Design review of the part built by this model. Coordinates are the model's own, in mm. A direction names the side the tool comes from. Round coordinates to 2 decimals unless told otherwise and drop trailing zeros. Order: outer loops, then holes, each group sorted by start corner. A loop starts at its lowest first (then second) coordinate and runs counter-clockwise, first axis right, second up. Notation, with made-up numbers: (-38.75, 43.5) - (1.25, 43.5) arc R19 cw to (1.25, 67.5) - close; hole circle Ø9 at (25.25, -39). An arc over 180 degrees is marked (long way). Write item = value, one per line.
from build123d import *

# Parameters (mm, degrees)
F0_W     = 6.35
F0_H     = 301.752
F1_DEPTH = 101.6
F3_DEPTH = 101.6
F5_DEPTH = 4.7625
F7_DEPTH = 4.7625
F8_W     = 127
F8_H     = 190.5
F9_DEPTH = 9.525
F11_D    = 11.1125


with BuildPart() as f1:
    # F0 (on Front) → F1 (new body, symmetric)
    with BuildSketch(Plane.XZ):
        Polygon((-19.05, -454.152), (0, -454.152), (0, 0), (-19.05, 0), (-19.05, -301.752), align=None)
        with Locations((-22.225, -150.876)):
            Rectangle(F0_W, F0_H)
    extrude(amount=F1_DEPTH, both=True)

    # F2 (on Front) → F3 (join, symmetric)
    with BuildSketch(Plane.XZ):
        Polygon((-158.75, 0), (0, 0), (298.45, 0), (298.45, 12.7), (-158.75, 12.7), align=None)
    extrude(amount=F3_DEPTH, both=True)

    # F4 (on Front) → F5 (join, symmetric)
    with BuildSketch(Plane.XZ):
        Polygon((-25.4, -127), (-25.4, 0), (-152.4, 0), (-152.4, -25.4), (-50.8, -127), align=None)
    extrude(amount=F5_DEPTH, both=True)

    # F6 (on Front) → F7 (join, symmetric)
    with BuildSketch(Plane.XZ):
        Polygon((292.1, 0), (0, 0), (0, -454.152), (25.4, -454.152), (292.1, -25.4), align=None)
    extrude(amount=F7_DEPTH, both=True)

    # F8 (on face) → F9 (join)
    with BuildSketch(Plane.XY.offset(12.7)):
        with Locations((-88.9, 0)):
            Rectangle(F8_W, F8_H)
        with Locations((228.6, 0)):
            Rectangle(F8_W, F8_H)
    extrude(amount=F9_DEPTH)

    # F11 (through all)
    with Locations(Plane.XY.offset(22.225)):
        with Locations((-127, 61.976), (-50.8, 61.976), (-127, -61.976), (-50.8, -61.976), (190.5, 61.976), (266.7, 61.976), (266.7, -61.976), (190.5, -61.976)):
            Hole(F11_D / 2)


solid = f1.part
Item 1: Take a section at D-D, the plane x = 102.5. State the section outline as (y, z) points.
Data:
outline = (-101.6, 0) - (-4.76, 0) - (-4.76, -330.2) - (4.76, -330.2) - (4.76, 0) - (101.6, 0) - (101.6, 12.7) - (-101.6, 12.7) - close
Item 2: Insertion check: P1, Ø10, axis at y = -73.5, z = -347, coming from the +X side; P2, Ø13, axis at x = 190.5, y = 61.976, coming from the -Z side; P3, Ø10.5, axis at x = 205.5, z = 19, coming from the -Y side. Each pin has a flat end and moves straight along its axis. Give the tip position at first contact, or say it passes through.
Data:
P1 = 0
P2 = 0
P3 = -95.25
Item 3: For faces 4 (the face through (-19.05, -1, -377)), 5 (the face through (-76, -4.762, -48)), 6 (the face through (194.595, 65.731, 10.957)), 7 (the face through (112, 4.762, -173)), list the 3-axis set-ups (+Z, -Z, +X, -X, +Y, -Y) from which the entire face can be reached by the end or side of a thin tool; tool diameter is ignored.
Data:
face_4 = -Z, -X, +Y, -Y
face_5 = -Z, -X, -Y
face_6 = +Z, -Z
face_7 = -Z, +X, +Y
Item 4: Take a section at B-B, the plane y = -36.5. State the section outline as (x, z) points (3 decimals).
Data:
outline = (-158.75, 0) - (-25.4, 0) - (-25.4, -301.752) - (-19.05, -301.752) - (-19.05, -454.152) - (0, -454.152) - (0, 0) - (298.45, 0) - (298.45, 12.7) - (292.1, 12.7) - (292.1, 22.225) - (165.1, 22.225) - (165.1, 12.7) - (-25.4, 12.7) - (-25.4, 22.225) - (-152.4, 22.225) - (-152.4, 12.7) - (-158.75, 12.7) - close
Item 5: Take a section at C-C, the plane z = -280. State the section outline as (x, y) points.
Data:
outline = (-25.4, -101.6) - (0, -101.6) - (0, -4.76) - (133.73, -4.76) - (133.73, 4.76) - (0, 4.76) - (0, 101.6) - (-25.4, 101.6) - close
Item 6: Take a section at A-A, the plane x = -127. Count the separate pieces of the cut face and the enclosed holes in it, and give its area (3 significant figures).
Data:
separate_pieces = 3
enclosed_holes = 0
area = 4,390 mm2
Item 7: For line 1 along Y through (x, z) = (266, 10); line 2 along Y through (x, z) = (-127, 6); line 3 along Z through (x, y) = (105, -68), list the stretches that pass through material, from the lowest coordinate up. Write a range as [from, to].
Data:
line_1 = [-101.6, -67.49], [-56.46, 56.46], [67.49, 101.6]
line_2 = [-101.6, -67.53], [-56.42, 56.42], [67.53, 101.6]
line_3 = [0, 12.7]
Item 8: The part is to be moulded in two halves that separate along Y. For faces 1 (the face through (-7, -1, -454.152)), 2 (the face through (-132.3, -60.31, 10.96)), 3 (the face through (112, -4.762, -173)), say which applies: +Y half, -Y half, draft (parallel to the pull), parting line (faces both ways), or undercut.
Data:
face_1 = draft
face_2 = undercut
face_3 = -Y half
